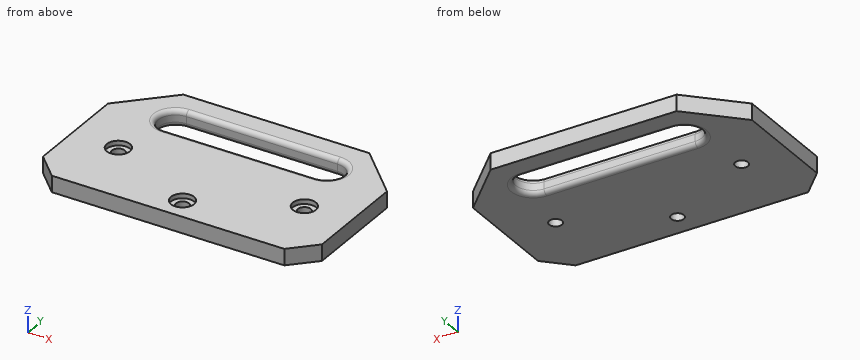
```python
from build123d import *

# Parameters (mm, degrees)
F0_W           = 120
F0_H           = 75
F1_DEPTH       = 7
F2_SIZE        = 20
F3_W           = 65
F3_H           = 0.0804045208
F4_DEPTH       = 25
F5_DEPTH       = 5
F6_SIZE        = 10
F7_R           = 2
F9_D           = 5.5
F9_CBORE_D     = 10
F9_CBORE_DEPTH = 2


with BuildPart() as f1:
    # F0 (on Top) → F1 (new body)
    with BuildSketch(Plane.XY):
        Rectangle(F0_W, F0_H)
    extrude(amount=F1_DEPTH)

    # F2
    f2_edges = [f1.edges().sort_by_distance(p)[0] for p in [
        (-60, 37.5, 3.5),
        (60, 37.5, 3.5),
    ]]
    chamfer(f2_edges, length=F2_SIZE)

    # F3 (on face) → F4 (cut)
    with BuildSketch(Plane.XY.offset(7)):
        with BuildLine():
            ThreePointArc((32.5, 12.5402022604), (40, 20.0402022604), (32.5, 27.5402022604))
            Line((32.5, 27.5402022604), (-32.5, 27.5402022604))
            ThreePointArc((-32.5, 27.5402022604), (-40, 20.0402022604), (-32.5, 12.5402022604))
            Line((-32.5, 12.5402022604), (32.5, 12.5402022604))
        make_face()
        with Locations((0, 20)):
            Rectangle(F3_W, F3_H, mode=Mode.SUBTRACT)
    extrude(amount=-F4_DEPTH, mode=Mode.SUBTRACT)

    # F5 (cut): a face of the model
    f5_faces = [f1.faces().sort_by_distance(p)[0] for p in [
        (0, 20.0402022604, 3.5),
    ]]
    extrude(f5_faces, amount=-F5_DEPTH, mode=Mode.SUBTRACT)

    # F6
    f6_edges = [f1.edges().sort_by_distance(p)[0] for p in [
        (-60, -37.5, 3.5),
        (60, -37.5, 3.5),
    ]]
    chamfer(f6_edges, length=F6_SIZE)

    # F7
    f7_edges = [f1.edges().sort_by_distance(p)[0] for p in [
        (40, 20.040202, 7),
        (40, 20.040202, 0),
    ]]
    fillet(f7_edges, radius=F7_R)

    # F9 (through all)
    with Locations(Plane.XY.offset(7)):
        with Locations((-40, -7.5), (0, -27.5), (40, -7.5)):
            CounterBoreHole(F9_D / 2, F9_CBORE_D / 2, F9_CBORE_DEPTH)


solid = f1.part
```
Read the model definition and answer for the solid it produces. Units are mm, in the model's axes. Give positions to 0.01 mm unless a question says otherwise; leave off trailing zeros. Order: outer loops, then holes, each group sorted by start corner. A loop starts at its lowest first (then second) coordinate and runs counter-clockwise, first axis right, second up.
(1) Find section A-A (x = 0). Give the vertices of the cut face in (y, z).
(2) Find section D-D (y = 31). Give the vertices of the cut face in (x, z).
(3) Find section C-C (x = -17). Give the vertices of the cut face in (y, z).
(4) Straight lines are drawn through the part: L1, parallel to Y at x = -31.5, z = 2; L2, parallel to Y at x = 0, z = 5.8; L3, parallel to Y at x = 6, z = 0.5. For each, find the intervals that lie inside material, in ascending order.
(5) Given pin 1 (16 mm diameter, centred on x = -40, y = -7.5, fed in from -Z); pin 2 (1.5 mm diameter, centred on y = -29, z = 5.5, fed in from -X), each flat-ended and moving along its own axis, determine where each tip first touches the part or whether it passes through.
(6) Find section B-B (y = -7.5). Give the vertices of the cut face in (x, z), plus the area to 3 significant figures.
Result sheet:
1. outline: (-37.5, 0) - (-30.25, 0) - (-30.25, 5) - (-32.5, 5) - (-32.5, 7) - (-37.5, 7) - close; (-24.75, 0) - (10.54, 0) arc R2 ccw to (12.54, 2) - (12.54, 5) arc R2 ccw to (10.54, 7) - (-22.5, 7) - (-22.5, 5) - (-24.75, 5) - close; (27.54, 2) arc R2 ccw to (29.54, 0) - (37.5, 0) - (37.5, 7) - (29.54, 7) arc R2 ccw to (27.54, 5) - close
2. outline: (-46.5, 0) - (46.5, 0) - (46.5, 7) - (-46.5, 7) - close
3. outline: (-37.5, 0) - (10.54, 0) arc R2 ccw to (12.54, 2) - (12.54, 5) arc R2 ccw to (10.54, 7) - (-37.5, 7) - close; (27.54, 2) arc R2 ccw to (29.54, 0) - (37.5, 0) - (37.5, 7) - (29.54, 7) arc R2 ccw to (27.54, 5) - close
4. L1: y = -37.5 to 12.54, 27.54 to 37.5
4. L2: y = -37.5 to -32.5, -22.5 to 12.37, 27.71 to 37.5
4. L3: y = -37.5 to 11.86, 28.22 to 37.5
5. pin 1: stops at z = 0
5. pin 2: stops at x = -59.25
6. outline: (-60, 0) - (-42.75, 0) - (-42.75, 5) - (-45, 5) - (-45, 7) - (-60, 7) - close; (-37.25, 0) - (37.25, 0) - (37.25, 5) - (35, 5) - (35, 7) - (-35, 7) - (-35, 5) - (-37.25, 5) - close; (42.75, 0) - (60, 0) - (60, 7) - (45, 7) - (45, 5) - (42.75, 5) - close
6. area: 745 mm2
